Study the drawing (mm; zero at the part's minimum x, y, z) and answer. A direction names the side the tool comes from. Coordinates: 2 decimals unless noted, no trailing zeros. Write each loop counter-clockwise with the first axis right and the second up, starting at its lowest first coordinate (ties: lowest second). Pieces come first, ordered by that corner, then holes. Notation, with made-up numbers: (41, 64) - (85, 64) arc R8 ccw to (85, 75) - close; hole circle Ø7 at (-24.75, 23). An arc over 180 degrees is marked (long way). One line per item, written item: value.
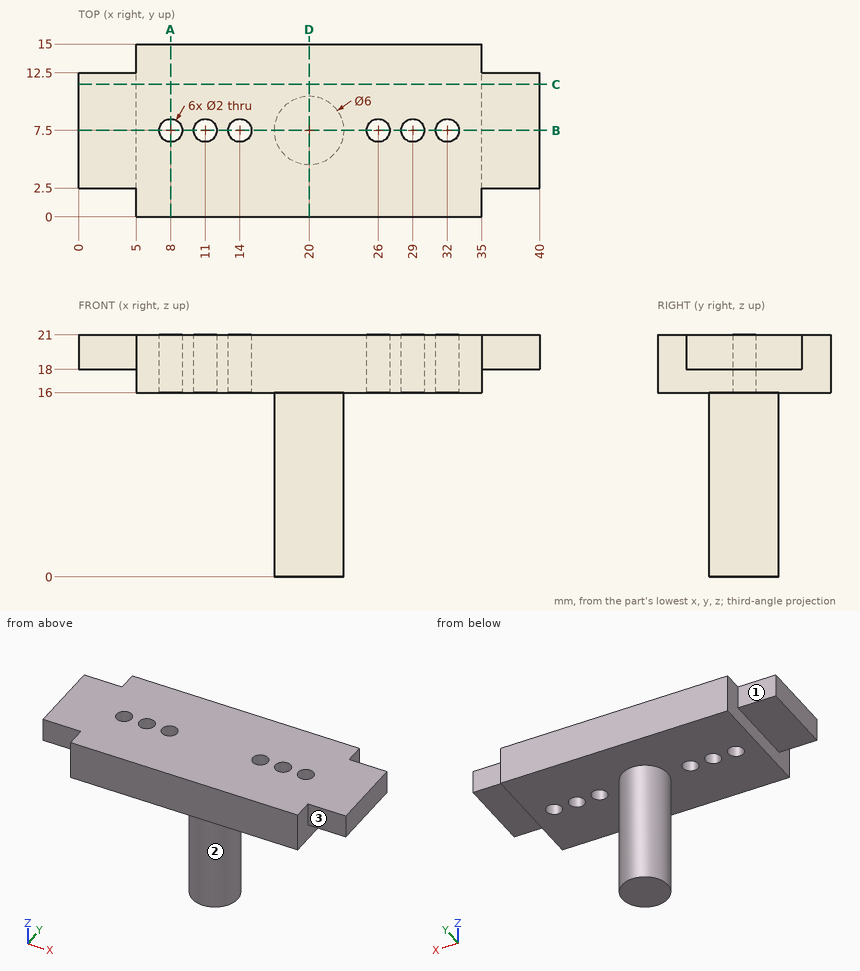
Item 1: Consider probe 1 along Y at (x, z) = (32, 17.25); probe 2 along Z at (x, y) = (9, 12.5); probe 3 along Z at (x, y) = (2.5, 5.5). Determine where each line is inside the solid, lowest interval first.
Evaluation:
probe 1: y = 0 to 6.5, 8.5 to 15
probe 2: z = 16 to 21
probe 3: z = 18 to 21
Item 2: Section A-A, the plane x = 8 is taken. Determine the outline of the cut face in (y, z).
Evaluation:
outline: (0, 16) - (6.5, 16) - (6.5, 21) - (0, 21) - close; (8.5, 16) - (15, 16) - (15, 21) - (8.5, 21) - close
Item 3: Section C-C, the plane y = 11.5 is taken. Determine the outline of the cut face in (x, z).
Evaluation:
outline: (0, 18) - (5, 18) - (5, 16) - (35, 16) - (35, 18) - (40, 18) - (40, 21) - (0, 21) - close
Item 4: Given pin 1 (1.2 mm diameter, centred on x = 26, y = 7.5, fed in from -Z); pin 2 (1 mm diameter, centred on y = 7.5, z = 14.5, fed in from -X); pin 3 (1.5 mm diameter, centred on x = 2.5, z = 19.5, fed in from +Y); pin 4 (4 mm diameter, centred on x = 1.5, y = 7.5, fed in from -Z), each flat-ended and moving along its own axis, determine where each tip first touches the part or whether it passes through.
Evaluation:
pin 1: passes through
pin 2: stops at x = 17
pin 3: stops at y = 12.5
pin 4: stops at z = 18
Item 5: Section B-B, the plane y = 7.5 is taken. Give the number of separate pieces and of enclosed holes in the cut face, then the cut area to 3 significant figures.
Evaluation:
separate pieces: 7
enclosed holes: 0
area: 216 mm2
Item 6: Section D-D, the plane x = 20 is taken. Determine the outline of the cut face in (y, z).
Evaluation:
outline: (0, 16) - (4.5, 16) - (4.5, 0) - (10.5, 0) - (10.5, 16) - (15, 16) - (15, 21) - (0, 21) - close
Item 7: Which of the six approach directions +Z, -Z, +X, -X, +Y, -Y give full straight-line access (tool end or side, diameter ignored) to the marked faces 1, 2 and 3?
Evaluation:
face 1: +Z, -Z, -X, +Y
face 2: -Z
face 3: +Z, -Z, +X, -Y
